Autodesk Inventor part; units mm, degrees
ref_plane "작업 평면1" through (0.95, 3.05, 0) normal (0, -1, 0) x (1, 0, 0)
ref_plane "YZ Plane" through (0, 0, 0) normal (1, 0, 0) x (0, 1, 0)
ref_plane "XZ Plane" through (0, 0, 0) normal (0, 1, 0) x (-1, 0, 0)
sketch "스케치1" plane through (0, 0, 0) normal (0, 0, 1) x (1, 0, 0)
  line L0 (4.6, 1.75) -> (2.95, 1.75)
  line L1 (1.75, 2.95) -> (1.75, 6.65)
  line L2 (-0.25, 6.65) -> (-0.25, 0.95)
  line L3 (0.95, -0.25) -> (4.6, -0.25)
  arc A0 (-0.25, 0.95) -> (0.95, -0.25) centre (0.95, 0.95) ccw
  line L4 (0.25, 6.65) -> (0.25, 0.95)
  arc A1 (0.25, 0.95) -> (0.95, 0.25) centre (0.95, 0.95) ccw
  line L5 (0.95, 0.25) -> (4.6, 0.25)
  arc A2 (1.75, 2.95) -> (2.95, 1.75) centre (2.95, 2.95) ccw
  line L6 (2.25, 6.65) -> (2.25, 2.95)
  arc A3 (2.25, 2.95) -> (2.95, 2.25) centre (2.95, 2.95) ccw
  line L7 (2.95, 2.25) -> (4.6, 2.25)
  line L8 (-0.25, 6.65) -> (0.25, 6.65)
  line L9 (1.75, 6.65) -> (2.25, 6.65)
  line L10 (4.6, 2.25) -> (4.6, 1.75)
  line L11 (4.6, 0.25) -> (4.6, -0.25)
  point P0 (0, 0)
  point P1 (1.75, 1.75)
  point P2 (-0.25, -0.25)
  dimension "d12" = 1.2
  dimension "d13" = 0.5
  dimension "d14" = 1.2
  dimension "d15" = 0.5
extrude "돌출1" add sketch "스케치1" along normal blind 0.5
ref_plane "작업 평면1" through (0.95, 3.05, 0) normal (0, -1, 0) x (1, 0, 0)
sketch "스케치2" plane through (0.95, 3.05, 0) normal (0, -1, 0) x (1, 0, 0)
  line L0 (-1.2, 0) -> (0, 0)
  line L1 (0, 0) -> (0, 0.5)
  line L2 (-1.2, 0.5) -> (0, 0.5)
  line L3 (-1.2, 0) -> (-1.2, 0.5)
  line L4 (0, 0.5) -> (3.65, 0.5)
  line L5 (0, 0) -> (0, 0.5)
  line L6 (0, 0) -> (3.65, 0)
  line L7 (0.94, 0.14) -> (1.16, 0.14)
  line L8 (0.94, 0.36) -> (0.94, 0.14)
  line L9 (1.16, 0.36) -> (0.94, 0.36)
  line L10 (1.16, 0.14) -> (1.16, 0.36)
  line L11 (-0.7, 0) -> (-1.2, 0)
  line L12 (-1.2, 0) -> (1.3, 0)
  line L13 (1.3, 0) -> (1.3, 0.5)
  line L14 (1.3, 0.5) -> (-1.2, 0.5)
  line L15 (-1.2, 0.5) -> (-1.2, 0)
  line L16 (-1.95, 1.25) -> (2.05, 1.25)
  line L17 (2.05, 1.25) -> (2.05, -0.75)
  line L18 (2.05, -0.75) -> (-1.95, -0.75)
  line L19 (-1.95, -0.75) -> (-1.95, 1.25)
  line L20 (-0.7, 0) -> (-0.7, 0.5)
  line L21 (-1.2, 0) -> (-1.2, 0.5)
  line L22 (-0.7, 0) -> (-1.2, 0)
  line L23 (-0.7, 0.5) -> (-1.2, 0.5)
  line L24 (3.65, 0) -> (3.65, 0.5)
  point P0 (-0.95, 0)
  dimension "d36" = 0.75
extrude "돌출2" add sketch "스케치2" against normal blind 2 contours L3 L2 L20 L0 | L0 L6 L17 L18 L19 L16 L4 L2 L3 | L20 L2 L1 L0 | L1 L4 L13 L6 | L13 L4 L17 L6 | L8 L9 L10 L7
chamfer "모따기7" distance 0.14 angle 70 4 edges at (0, 6.65, 0.5) (-0.25, 6.65, 0.25) (0, 6.65, 0) (0.25, 6.65, 0.25) measured on face at (0.0833, 6.65, 0.1667)
chamfer "모따기8" distance 0.14 angle 70 4 edges at (1.75, 6.65, 0.25) (2, 6.65, 0) (2.25, 6.65, 0.25) (2, 6.65, 0.5) measured on face at (2.0833, 6.65, 0.1667)
chamfer "모따기9" distance 0.14 angle 70 4 edges at (4.6, 2, 0.5) (4.6, 2.25, 0.25) (4.6, 2, 0) (4.6, 1.75, 0.25) measured on face at (4.6, 1.9167, 0.1667)
chamfer "모따기10" distance 0.14 angle 70 4 edges at (4.6, 0.25, 0.25) (4.6, 0, 0.5) (4.6, 0, 0) (4.6, -0.25, 0.25) measured on face at (4.6, -0.0833, 0.1667)
chamfer "모따기11" distance 0.5 angle 45 4 edges at (-1, 4.05, 1.25) (3, 4.05, 1.25) (3, 4.05, -0.75) (-1, 4.05, -0.75)
pattern_linear "직사각형 패턴1" count 2 spacing 2 along (0, 0, 1) of "돌출1", "돌출2", "모따기7", "모따기8", "모따기9", "모따기10", "모따기11"
ref_plane "작업 평면2" through (0.95, 3.05, 2) normal (0, -1, 0) x (1, 0, 0)
properties part number "2pin_header"
Input: part model. Units: mm. Frame: model coordinates. A direction names the side the tool comes from. Coordinates: 2 decimals unless noted, no trailing zeros. Order: outer loops, then holes, each group sorted by start corner. A loop starts at its lowest first (then second) coordinate and runs counter-clockwise, first axis right, second up. Notation, with made-up numbers: M 82,48.5 L 99,48.5 A10 ccw 99,59.5 Z; hole C 64.5,-25 d9. An arc over 180 degrees is marked long. Write item = value, one per line. Start each with the question number.
(1) Reachability of faces 1 (the flat face through (1, 0, 0.5)), 2 (the flat face through (3, 2, 0)), 3 (the flat face through (1, 4, 3.25)), 4 (the flat face through (3, 4, 2)), 5 (the flat face through (1, 0, 2.5)) from +Z, -Z, +X, -X, +Y, -Y: full face, straight path, thin tool, end or side. Return the list, or none.
(2) Pull-direction query (X, two-part tool) for faces 6 (the cylindrical face through (2.111, 2.092, 0.246)), 7 (the flat face through (3, 2, 2.5)), 8 (the cylindrical face through (2.111, 2.092, 2.246)), 9 (the flat face through (-1, 4, 2)); classes: released by +X, released by -X, zero draft, split by the parting line, or undercut.
(3) Line query: line 1 along Z through (x, y) = (-0.2, 2); line 2 along Y through (x, z) = (2.75, -0.15); line 3 along X through (y, z) = (3.25, -0.1). Output: solid intervals per line, ascending. Write a range as [from, to].
(4) Section A-A on x = 3.9. Output: boundary loops of the cut face in (y, z).
(5) First-contact query: P1, Ø1.6, axis at x = 1, y = 1.5, coming from the -Z side; P2, Ø0.6, axis at x = 3, y = 2.5, coming from the +Z side; P3, Ø1.4, axis at x = 3, y = 2.5, coming from the -Z side. Flat tips, straight axial feed; report the tip coordinate or a pass-through.
(6) Section B-B on y = 1.25. Output: boundary loops of the cut face in (x, z), and give its area (3 significant figures).
Result set:
q1.face_1 = +X, -X, -Y
q1.face_2 = -Z, +X, -X, -Y
q1.face_3 = +Z, +X, -X, +Y, -Y
q1.face_4 = +Z, -Z, +X, +Y
q1.face_5 = +Z, +X, -X, -Y
q2.face_6 = undercut
q2.face_7 = zero draft
q2.face_8 = undercut
q2.face_9 = released by -X
q3.line_1 = [0, 0.5], [2, 2.5]
q3.line_2 = [3.05, 5.05]
q3.line_3 = [-1, 3]
q4.outline = M -0.25,0 L 0.25,0 L 0.25,0.5 L -0.25,0.5 Z; M -0.25,2 L 0.25,2 L 0.25,2.5 L -0.25,2.5 Z; M 1.75,0 L 2.25,0 L 2.25,0.5 L 1.75,0.5 Z; M 1.75,2 L 2.25,2 L 2.25,2.5 L 1.75,2.5 Z
q5.P1 = 0
q5.P2 = 2.5
q5.P3 = -0.68
q6.outline = M -0.25,0 L 0.25,0 L 0.25,0.5 L -0.25,0.5 Z; M -0.25,2 L 0.25,2 L 0.25,2.5 L -0.25,2.5 Z
q6.area = 0.500 mm²
